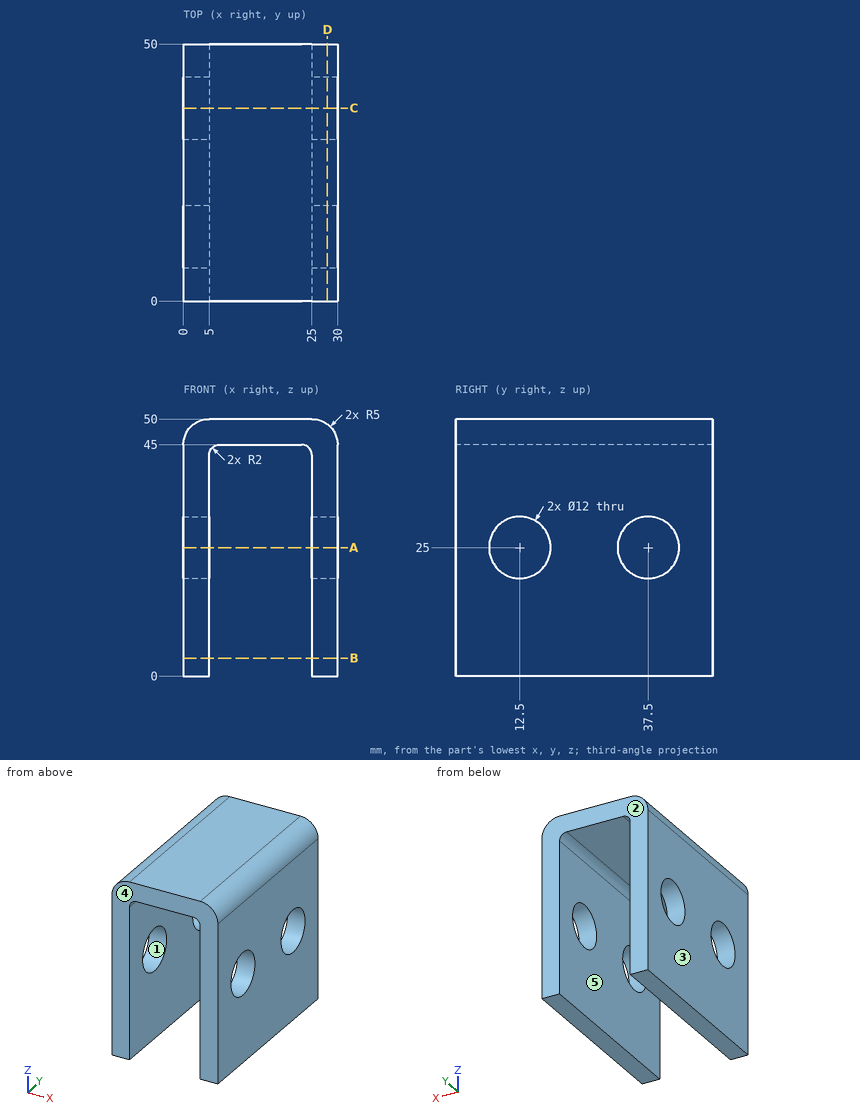
Check sheet for the drawn part. Datum: minimum x, y, z corner. Units: mm. A direction names the side the tool comes from. Round coordinates to 2 decimals unless told otherwise and drop trailing zeros. Order: outer loops, then holes, each group sorted by start corner. A loop starts at its lowest first (then second) coordinate and runs counter-clockwise, first axis right, second up. Notation, with made-up numbers: M 80,81 L 127,81 A24 cw 127,91 Z; hole C 35,-3 d9. An arc over 180 degrees is marked long. Write each question's results on one line, items separated by ' | '. Start each with the question number.
1. Cross-section at C-C on y = 37.5. Record the boundary of the cut face in (x, z), plus the area to 3 significant figures.
2. Set-up check for the marked faces 4 and 5: record each of +Z, -Z, +X, -X, +Y, -Y from which the full face is reachable in a straight line by a thin tool's end or side.
3. Cross-section at D-D on x = 28. Record the boundary of the cut face in (y, z), plus the area to 3 significant figures.
4. Cross-section at B-B on z = 3.5. Record the boundary of the cut face in (x, y), plus the area to 3 significant figures.
5. Draft check along Y on the marked faces 1, 2 and 3. Enter one of: pulls with the +Y half, pulls with the -Y half, needs draft (parallel to the pull), parting line crosses it, or undercut.
6. Go/stop test with a flat-tipped pin: P1, Ø17.5, axis at x = 18, y = 27, coming from the -Z side. Record where the tip stops, or that it passes through.
7. Cross-section at A-A on z = 25. Record the boundary of the cut face in (x, y).
8. Material ranges on L1, parallel to X at y = 46, z = 13.5; L2, parallel to Z at x = 13.75, y = 18; L3, parallel to Z at x = 1.5, y = 7, recorded low to high. Write a range as from..to.
Resolved:
1) outline: M 0,0 L 5,0 L 5,19 L 0,19 Z; M 0,31 L 5,31 L 5,43 A2 cw 7,45 L 23,45 A2 cw 25,43 L 25,31 L 30,31 L 30,45 A5 ccw 25,50 L 5,50 A5 ccw 0,45 Z; M 25,0 L 30,0 L 30,19 L 25,19 Z | area: 471 mm2
2) face 4: +Z, -Z, +X, -X, -Y | face 5: -Z, +Y, -Y
3) outline: M 0,0 L 50,0 L 50,49 L 0,49 Z; hole C 12.5,25 d12; hole C 37.5,25 d12 | area: 2,220 mm2
4) outline: M 0,0 L 5,0 L 5,50 L 0,50 Z; M 25,0 L 30,0 L 30,50 L 25,50 Z | area: 500 mm2
5) face 1: undercut | face 2: pulls with the +Y half | face 3: needs draft
6) P1: z = 0
7) outline: M 0,0 L 5,0 L 5,6.5 L 0,6.5 Z; M 0,18.5 L 5,18.5 L 5,31.5 L 0,31.5 Z; M 0,43.5 L 5,43.5 L 5,50 L 0,50 Z; M 25,0 L 30,0 L 30,6.5 L 25,6.5 Z; M 25,18.5 L 30,18.5 L 30,31.5 L 25,31.5 Z; M 25,43.5 L 30,43.5 L 30,50 L 25,50 Z
8) L1: 0..5, 25..30 | L2: 45..50 | L3: 0..22.6, 27.4..48.57
